Can you work these out from the model? Positions are in its coordinate system, mm. A direction names the side the tool comes from. Give positions to 0.01 mm unless a question says otherwise; leave off trailing zeros. Write each loop counter-clockwise with the first axis right and the second up, starting at its lowest first coordinate (ties: lowest second). Pieces come first, ordered by that corner, then holes.
```python
from build123d import *

# Parameters (mm, degrees)
F1_DEPTH = 63.5
F0_W     = 27.836654
F0_H     = 19.05
F2_DEPTH = 25.4
F3_DEPTH = 3.3655
F4_R     = 5.08


with BuildPart() as f1:
    # F0 (on Front) → F1 (new body, symmetric)
    with BuildSketch(Plane.XZ):
        Polygon((22.225, 9.525), (-41.275, 9.525), (-41.275, -9.525), (41.275, -9.525), (41.275, 9.525), align=None)
    extrude(amount=F1_DEPTH, both=True)

    # F0 (on Front) → F2 (join, symmetric)
    with BuildSketch(Plane.XZ):
        with BuildLine():
            Line((22.225, 25.90316), (22.225, 9.525))
            Line((22.225, 9.525), (41.275, 9.525))
            Line((41.275, 9.525), (41.275, 26.260685))
            ThreePointArc((41.275, 26.260685), (45.648964, 37.960944), (57.132766, 42.8752))
            Line((57.132766, 42.8752), (60.325, 42.8752))
            Line((60.325, 42.8752), (60.325, 61.9252))
            Line((60.325, 61.9252), (57.132766, 61.9252))
            add(Edge.make_bspline(
                [(57.132766, 61.9252), (56.532725, 61.915433), (55.926231, 61.899604), (55.313651, 61.877792)],
                knots=[0, 0, 0, 0, 1.808043, 1.808043, 1.808043, 1.808043], degree=3))
            ThreePointArc((55.313651, 61.877792), (31.427523, 50.643299), (22.225, 25.90316))
        make_face()
        with Locations((74.243327, 52.4002)):
            Rectangle(F0_W, F0_H)
    extrude(amount=F2_DEPTH, both=True)

    # F0 (on Front) → F3 (join, symmetric)
    with BuildSketch(Plane.XZ):
        with BuildLine():
            add(Edge.make_bspline(
                [(55.313651, 61.877792), (18.152726, 60.55465), (-41.403137, 37.216185), (-41.275, 9.525)],
                knots=[1.808043, 1.808043, 1.808043, 1.808043, 111.489324, 111.489324, 111.489324, 111.489324], degree=3))
            Line((-41.275, 9.525), (22.225, 9.525))
            Line((22.225, 9.525), (22.225, 25.90316))
            ThreePointArc((22.225, 25.90316), (31.427523, 50.643299), (55.313651, 61.877792))
        make_face()
    extrude(amount=F3_DEPTH, both=True)

    # F4
    f4_edges = [f1.edges().sort_by_distance(p)[0] for p in [
        (41.275, -63.5, 0),
        (-41.275, -63.5, 0),
        (41.275, 63.5, 0),
        (-41.275, 63.5, 0),
    ]]
    fillet(f4_edges, radius=F4_R)

    # F0 (on Front) → F5 (revolve)
    with BuildSketch(Plane.XZ):
        Polygon((88.161654, 66.675), (88.161654, 61.9252), (88.161654, 42.8752), (88.161654, 38.1), (111.125, 38.1), (111.125, 66.675), align=None)
    revolve(axis=Axis((88.161654, 0, 52.4002), (0, 0, 1)))


solid = f1.part
```
1) Please list where these lines run through material, in increasing order: L1, parallel to Z at x = -1, y = 15.5 (3 decimals); L2, parallel to Y at x = 54, z = 45; L3, parallel to Y at x = 23, z = 51.
Values follow:
L1: z = -9.525 to 9.525
L2: y = -25.4 to 25.4
L3: y = -3.37 to 3.37
2) For faces 4 (the face through (22.225, 14, 18)), 5 (the face through (47, 25.4, 42)), 6 (the face through (88, 0, 38.1)), 7 (the face through (22.225, -15, 18)), which set-ups out of +Z, -Z, +X, -X, +Y, -Y let a thin tool reach every point of the face, with its end or its side?
Values follow:
face 4: +Z, -X, +Y
face 5: +Z, +X, -X, +Y
face 6: -Z, +X, +Y, -Y
face 7: +Z, -X, -Y
3) For pin 1 Ø4 at (x, y) = (71, -8) entering from -Z; pin 2 Ø5 at (y, z) = (25.5, 39.5) entering from -X; pin 3 Ø8 at (x, z) = (37.5, 32) entering from +Y, each with a flat end and sliding along its axis, tell me the tip position at first contact or that it passes through.
Values follow:
pin 1: stops at z = 38.1
pin 2: stops at x = 23.67
pin 3: stops at y = 25.4
4) If we mould it in two halves opening along X, with no side actions, what happens to faces 1 (the face through (45.5, -0.4, 37.8)), 2 (the face through (31.686, -14.537, 50.921)), 3 (the face through (1, 33, 9.525))? For each: +X half, -X half, draft (parallel to the pull), parting line (faces both ways), or undercut.
Values follow:
face 1: undercut
face 2: -X half
face 3: draft
5) Suppose I cut it at A-A on y = -35. Write out the boundary of the cut face in (x, z) (3 decimals), plus the area to 3 significant figures.
Values follow:
outline: (-41.275, -9.525) - (41.275, -9.525) - (41.275, 9.525) - (-41.275, 9.525) - close
area: 1,570 mm2
6) Suppose I cut it at B-B on x = 59.5. Write out the boundary of the cut face in (y, z).
Values follow:
outline: (-25.4, 42.88) - (25.4, 42.88) - (25.4, 61.93) - (-25.4, 61.93) - close
